Verification items for the finished model (mm, model axes). A direction names the side the tool comes from. Coordinates: 2 decimals unless noted, no trailing zeros. Loops run counter-clockwise (first coordinate to the right, second up) from the corner with the lowest first, then second, coordinate; pieces in that order, holes last. Notation, with made-up numbers: (30, -14.75) - (76, -14.75) arc R22 cw to (76, 3.25) - close; hole circle Ø7 at (52.25, -17). An arc over 180 degrees is marked (long way). One line per item, written item: value. Start each with the question number.
(1) Section check B-B (z = -57). Record the boundary of the cut face in (x, y), plus the area to 3 significant figures.
(2) Section check C-C (x = 151.5). Record the boundary of the cut face in (y, z).
(3) Thickness scan on probe 1 along X at (y, z) = (4, -19); probe 2 along Z at (x, y) = (36.5, 3). Record the ranges inside material, lowest first. Write a range as [from, to].
(4) Set-up check for faces 1 (the face through (70, 15, -69)), 2 (the face through (109, 0, -65)): record each of +Z, -Z, +X, -X, +Y, -Y from which the full face is reachable in a straight line by a thin tool's end or side.
(5) Section check A-A (y = -0.5). Record the boundary of the cut face in (x, z), plus the area to 3 significant figures.
(6) Gauge pin test, flat ends, axial feed: P1, Ø9, axis at y = -6, z = -31, coming from the +X side; P2, Ø5, axis at x = 117.5, y = -2.5, coming from the +Z side. Record the tip position at first contact, or that the pin passes through.
```python
from build123d import *

# Parameters (mm, degrees)
SKETCH1_W = 30
SKETCH1_H = 30


with BuildPart() as part:
    # Sweep1: sweep along a path in Sketch2
    with BuildLine(Plane(origin=(0, 0, 0), x_dir=(1, 0, 0), z_dir=(0, 1, 0))) as sweep1_path:
        Line((0, 0), (0, 80))
        Line((0, 80), (200, 80))
    # Sketch1 → Sweep1 (sweep)
    with BuildSketch(Plane.XY):
        Rectangle(SKETCH1_W, SKETCH1_H)
    sweep(path=sweep1_path.line, transition=Transition.RIGHT)


solid = part.part
```
Responses:
1. outline: (-15, -15) - (15, -15) - (15, 15) - (-15, 15) - close
1. area: 900 mm²
2. outline: (-15, -95) - (15, -95) - (15, -65) - (-15, -65) - close
3. probe 1: x = [-15, 15]
3. probe 2: z = [-95, -65]
4. face 1: +Z, -Z, +X, -X, +Y
4. face 2: +Z, +X, +Y, -Y
5. outline: (-15, -95) - (200, -95) - (200, -65) - (15, -65) - (15, 0) - (-15, 0) - close
5. area: 8,400 mm²
6. P1: stops at x = 15
6. P2: stops at z = -65
